```python
from build123d import *

# Parameters (mm, degrees)
SKETCH1_R           = 17.5
BOSS_EXTRUDE1_DEPTH = 2
SKETCH2_R           = 17.5
BOSS_EXTRUDE2_DEPTH = 38
SKETCH3_W           = 4
SKETCH3_H           = 6
CUT_EXTRUDE1_DEPTH  = 46.348649373
SKETCH4_W           = 4
SKETCH4_H           = 6
CUT_EXTRUDE2_DEPTH  = 48.418350878


with BuildPart() as part:
    # Sketch1 → Boss-Extrude1 (new body)
    with BuildSketch(Plane.XY):
        Circle(SKETCH1_R)
    extrude(amount=BOSS_EXTRUDE1_DEPTH)

    # Sketch2 → Boss-Extrude2 (add)
    with BuildSketch(Plane.XY.offset(2)):
        Circle(SKETCH2_R)
        with BuildLine():
            Line((-1, 15.467708298), (-1, -15.467708298))
            ThreePointArc((-1, -15.467708298), (-15.5, 0), (-1, 15.467708298))
        make_face(mode=Mode.SUBTRACT)
        with BuildLine():
            Line((1, 15.467708298), (1, -15.467708298))
            ThreePointArc((1, -15.467708298), (15.5, 0), (1, 15.467708298))
        make_face(mode=Mode.SUBTRACT)
    extrude(amount=BOSS_EXTRUDE2_DEPTH)

    # Sketch3 → Cut-Extrude1 (cut, through all)
    with BuildSketch(Plane.XY.offset(2)):
        with Locations((7, 0)):
            Rectangle(SKETCH3_W, SKETCH3_H)
        with Locations((-7, 0)):
            Rectangle(SKETCH3_W, SKETCH3_H)
    extrude(amount=-CUT_EXTRUDE1_DEPTH, mode=Mode.SUBTRACT)

    # Sketch4 → Cut-Extrude2 (cut, through all)
    with BuildSketch(Plane.ZY.offset(1)):
        with Locations((7, 0)):
            Rectangle(SKETCH4_W, SKETCH4_H)
    cut_extrude2 = extrude(amount=CUT_EXTRUDE2_DEPTH, mode=Mode.SUBTRACT)

    # Mirror1: Cut-Extrude2 across plane
    add(cut_extrude2.mirror(Plane(origin=(0, 0, 0), x_dir=(0, 0, 1), z_dir=(1, 0, 0))), mode=Mode.SUBTRACT)


solid = part.part
```
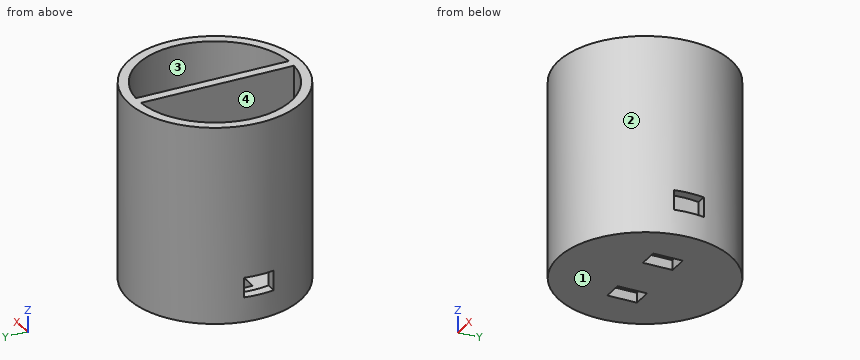
Work out the finished part from the listing and answer in its coordinate system (mm). Face numbers are marked on the shaded views. Coordinates: 2 decimals unless noted, no trailing zeros. Loops run counter-clockwise (first coordinate to the right, second up) from the corner with the lowest first, then second, coordinate; pieces in that order, holes last. Notation, with made-up numbers: (20, 85.25) - (31, 85.25) arc R8 cw to (31, 91.25) - close; hole circle Ø10 at (17, 88.5). An arc over 180 degrees is marked (long way). Use a Markdown table: item, result.
Item 1: Find section D-D, the plane y = 4. Determine the outline of the cut face in (x, z).
Evaluation:
| item | result |
|---|---|
| outline | (-17.04, 0) - (17.04, 0) - (17.04, 40) - (14.97, 40) - (14.97, 2) - (1, 2) - (1, 40) - (-1, 40) - (-1, 2) - (-14.97, 2) - (-14.97, 40) - (-17.04, 40) - close |
Item 2: Consider probe 1 along X at (y, z) = (-3, 12.5); probe 2 along X at (y, z) = (-12.5, 32.5); probe 3 along Y at (x, z) = (3, 28). Determine where each line is inside the solid, lowest interval first. Write a range as from..to.
Evaluation:
| item | result |
|---|---|
| probe 1 | x = -17.24..-15.21, -1..1, 15.21..17.24 |
| probe 2 | x = -12.25..-9.17, -1..1, 9.17..12.25 |
| probe 3 | y = -17.24..-15.21, 15.21..17.24 |
Item 3: Find section A-A, the plane y = 0. Determine the outline of the cut face in (x, z), and give its area (3 significant figures).
Evaluation:
| item | result |
|---|---|
| outline | (-17.5, 0) - (-9, 0) - (-9, 2) - (-15.5, 2) - (-15.5, 5) - (-17.5, 5) - close; (-17.5, 9) - (-15.5, 9) - (-15.5, 40) - (-17.5, 40) - close; (-5, 0) - (5, 0) - (5, 2) - (1, 2) - (1, 40) - (-1, 40) - (-1, 2) - (-5, 2) - close; (9, 0) - (17.5, 0) - (17.5, 5) - (15.5, 5) - (15.5, 2) - (9, 2) - close; (15.5, 9) - (17.5, 9) - (17.5, 40) - (15.5, 40) - close |
| area | 266 mm2 |
Item 4: The mould has two halves that part along Y. Classify the marked faces 1, 2, 3 and 4: +Y half, -Y half, draft (parallel to the pull), parting line (faces both ways), or undercut.
Evaluation:
| item | result |
|---|---|
| face 1 | draft |
| face 2 | parting line |
| face 3 | undercut |
| face 4 | undercut |
Item 5: Find section B-B, the plane z = 28. Determine the outline of the cut face in (x, y).
Evaluation:
| item | result |
|---|---|
| outline | circle Ø35 at (0, 0); hole (-1, -15.47) - (-1, 15.47) arc R15.5 ccw to start; hole (1, -15.47) arc R15.5 ccw to (1, 15.47) - close |
Item 6: Find section C-C, the plane x = -12.5. Determine the outline of the cut face in (y, z).
Evaluation:
| item | result |
|---|---|
| outline | (-12.25, 0) - (12.25, 0) - (12.25, 40) - (9.17, 40) - (9.17, 2) - (-9.17, 2) - (-9.17, 40) - (-12.25, 40) - close |
Item 7: Given pin 1 Ø4 at (y, z) = (7, 33) entering from +X; pin 2 Ø2 at (x, z) = (-7.5, 1) entering from -Y; pin 3 Ø0.6 at (x, z) = (16, 8) entering from -Y, each flat-ended and moving along its own axis, determine where each tip first touches the part or whether it passes through.
Evaluation:
| item | result |
|---|---|
| pin 1 | stops at x = 16.77 |
| pin 2 | stops at y = -16.25 |
| pin 3 | stops at y = -7.73 |
